Autodesk Inventor part; units mm, degrees
ref_plane "YZ Plane" through (0, 0, 0) normal (1, 0, 0) x (0, 1, 0)
ref_plane "XZ Plane" through (0, 0, 0) normal (0, 1, 0) x (-1, 0, 0)
ref_plane "XY Plane" through (0, 0, 0) normal (0, 0, 1) x (1, 0, 0)
sketch "Sketch1" plane through (0, 0, 0) normal (0, 0, 1) x (1, 0, 0)
  line L0 (0, 0) -> (10.795, 0)
  line L1 (10.795, 0) -> (10.795, 4.7625)
  line L2 (0, 0) -> (0, 4.7625)
  arc A0 (0, 4.7625) -> (10.795, 4.7625) centre (5.3975, 55.2749) ccw
  dimension "d0" = 50.8
  dimension "d1" = 10.795
  dimension "d2" = 4.7625
extrude "Extrusion1" add sketch "Sketch1" along normal blind 114.3
sketch "Sketch2" plane through (0, 0, 114.3) normal (0, 0, 1) x (1, 0, 0)
  arc A0 (0, 4.7625) -> (10.795, 4.7625) centre (5.3975, 55.2749) ccw
  line L0 (3.0162, 4.5308) -> (7.7787, 4.5308)
  line L1 (7.7787, 4.5308) -> (7.7787, 1.3558)
  line L2 (7.7787, 1.3558) -> (3.0162, 1.3558)
  line L3 (3.0162, 1.3558) -> (3.0162, 4.5308)
  point P0 (0, 0)
  point P1 (5.3975, 4.5308)
  point P2 (5.3975, 4.4749)
  dimension "d5" = 4.7625
  dimension "d6" = 3.175
extrude "Extrusion2" cut sketch "Sketch2" against normal through all contours A0 L1 L2 L3
chamfer "Chamfer2" distance 3.175 distance2 2.286 1 edges at (0, 0, 57.15) measured on face at (0, 3.175, 38.1)
chamfer "Chamfer3" distance 2.286 distance2 3.175 1 edges at (10.795, 0, 57.15) measured on face at (5.1223, 0, 38.1)
chamfer "Chamfer6" distance 4.7498 angle 45 1 edges at (5.3975, 0, 114.3)
properties part number "WireGuideToMiniSubExtender" material "ABS Plastic"
Source: CAD feature listing. Evaluate the final solid. Frame: model axes, mm. A direction names the side the tool comes from. Coordinates: 2 decimals unless noted, no trailing zeros. Order: outer loops, then holes, each group sorted by start corner. A loop starts at its lowest first (then second) coordinate and runs counter-clockwise, first axis right, second up. Notation, with made-up numbers: (-20.75, 34.25) - (-11.75, 34.25) arc R24 cw to (-11.75, 55.25) - close; hole circle Ø10 at (62, -26.75). An arc over 180 degrees is marked (long way). One line per item, written item: value.
1) Cut plane B-B on x = 4.5. Output: boundary loops of the cut face in (y, z), plus the area to 3 significant figures.
Computed values:
outline: (0, 0) - (1.36, 0) - (1.36, 110.91) - (0, 109.55) - close
area: 149 mm^2
2) Contact query for flat-ended pins moving along their axis: pin 1 (1 mm diameter, centred on x = 2.5, y = 4, fed in from +Z); pin 2 (1.4 mm diameter, centred on x = 6.5, z = 78, fed in from +Y). Output: stop coordinate, or through.
Computed values:
pin 1: stops at z = 114.05
pin 2: stops at y = 1.36
3) Reachability of faces 1 (the face through (1.159, 1.565, 55.574)), 2 (the face through (9.31, 4.626, 56.35)) from +Z, -Z, +X, -X, +Y, -Y: full face, straight path, thin tool, end or side. Return the list, or none.
Computed values:
face 1: +Z, -Z, -X, -Y
face 2: +Z, -Z, +Y
4) Ray query, line 1 (X direction, y = 3.65, z = 86.5) (3 decimals); line 2 (X direction, y = 1.85, z = 90.5); line 3 (Y direction, x = 6, z = 91.5). Return the intervals inside material, ascending. Write a range as [from, to].
Computed values:
line 1: x = [0, 3.016], [7.779, 10.795]
line 2: x = [0.95, 3.02], [7.78, 9.84]
line 3: y = [0, 1.36]
5) Cut plane A-A on z = 76. Output: boundary loops of the cut face in (x, y) (1 decimal).
Computed values:
outline: (0, 3.2) - (2.3, 0) - (8.5, 0) - (10.8, 3.2) - (10.8, 4.8) arc R50.8 cw to (7.8, 4.5) - (7.8, 1.4) - (3, 1.4) - (3, 4.5) arc R50.8 cw to (0, 4.8) - close
